The listing builds one solid part. Answer for the finished solid, in the listing's coordinates (mm). A direction names the side the tool comes from. Round coordinates to 2 decimals unless told otherwise and drop trailing zeros. Loops run counter-clockwise (first coordinate to the right, second up) from the corner with the lowest first, then second, coordinate; pieces in that order, holes last. Notation, with made-up numbers: (12.25, 41.25) -> (57.25, 41.25) arc R15 ccw to (57.25, 50.25) -> close; hole circle Ø11 at (-33, 11). An arc over 180 degrees is marked (long way). Use a Markdown table: item, result. Add a question column.
Q1. Consider line 1 (X direction, y = 0.5, z = -180); line 2 (X direction, y = 2.4, z = -20); line 3 (X direction, y = 1.65, z = -105). Determine where each line is inside the solid, lowest interval first.
Q2. Section C-C on x = 42.5 is taken. Give the vertices of the cut face in (y, z), then the cut area to 3 significant figures.
Q3. Section D-D on y = -1.5 is taken. Give the vertices of the cut face in (x, z), then the cut area to 3 significant figures.
Q4. Section A-A on z = -132.5 is taken. Give the vertices of the cut face in (x, y).
Q5. For a pull along X with two mould halves and no side action, classify faces 1 (the flat face through (0, 2, -96)), 2 (the cylindrical face through (117.6, 2, -170)) as released by +X, released by -X, zero draft, split by the parting line, or undercut.
Q6. Which of the six approach directions +Z, -Z, +X, -X, +Y, -Y give full straight-line access (tool end or side, diameter ignored) to faces 3 (the cylindrical face through (10, 2, -150)), 4 (the cylindrical face through (165, 2, -10))?
Q7. Given pin 1 Ø2 at (x, y) = (136, -2) entering from -Z, flat-ended and moving along its own axis, determine where the tip first touches the part or whether it passes through.
Q8. Section B-B on x = 115 is taken. Give the vertices of the cut face in (y, z).
from build123d import *

# Parameters (mm, degrees)
SKETCH1_W           = 200
SKETCH1_H           = 190
BOSS_EXTRUDE1_DEPTH = 4
SKETCH3_R           = 50
CUT_EXTRUDE5_DEPTH  = 10
SKETCH4_W           = 200
SKETCH4_H           = 4
BOSS_EXTRUDE2_DEPTH = 4
SKETCH_1_R          = 8
CUT_EXTRUDE_1_DEPTH = 10


with BuildPart() as part:
    # Sketch1 → Boss-Extrude1 (new body)
    with BuildSketch(Plane(origin=(0, 0, 0), x_dir=(1, 0, 0), z_dir=(0, 1, 0))):
        with Locations((100, 95)):
            Rectangle(SKETCH1_W, SKETCH1_H)
    extrude(amount=BOSS_EXTRUDE1_DEPTH)

    # Sketch3 → Cut-Extrude5 (cut)
    with BuildSketch(Plane(origin=(0, 4, 0), x_dir=(1, 0, 0), z_dir=(0, 1, 0))):
        with BuildLine():
            Line((30, 15), (20.262068061, 15))
            ThreePointArc((20.262068061, 15), (16.735494747, 16.716132106), (15, 20.233217082))
            Line((15, 20.233217082), (15, 30))
            ThreePointArc((15, 30), (10, 35), (5, 30))
            Line((5, 30), (5, 20.194837008))
            ThreePointArc((5, 20.194837008), (4.997925704, 19.868737095), (5.017113168, 19.54319555))
            ThreePointArc((5.017113168, 19.54319555), (9.654794827, 9.654664453), (19.545086076, 5.020737673))
            ThreePointArc((19.545086076, 5.020737673), (19.772306824, 5.005187109), (20, 5))
            Line((20, 5), (30, 5))
            ThreePointArc((30, 5), (35, 10), (30, 15))
        make_face()
        with BuildLine():
            Line((5, 90), (5, 50))
            ThreePointArc((5, 50), (10, 45), (15, 50))
            Line((15, 50), (15, 90))
            ThreePointArc((15, 90), (10, 95), (5, 90))
        make_face()
        with BuildLine():
            Line((70, 15), (50, 15))
            ThreePointArc((50, 15), (45, 10), (50, 5))
            Line((50, 5), (70, 5))
            ThreePointArc((70, 5), (75, 10), (70, 15))
        make_face()
        with BuildLine():
            ThreePointArc((185, 50), (190, 45), (195, 50))
            Line((195, 50), (195, 90))
            ThreePointArc((195, 90), (190, 95), (185, 90))
            Line((185, 90), (185, 50))
        make_face()
        with BuildLine():
            ThreePointArc((185, 20.233217082), (183.264505253, 16.716132106), (179.737931939, 15))
            Line((179.737931939, 15), (170, 15))
            ThreePointArc((170, 15), (165, 10), (170, 5))
            Line((170, 5), (180, 5))
            ThreePointArc((180, 5), (180.227693176, 5.005187109), (180.454913924, 5.020737673))
            ThreePointArc((180.454913924, 5.020737673), (190.345205173, 9.654664453), (194.982886832, 19.54319555))
            ThreePointArc((194.982886832, 19.54319555), (195.002074296, 19.868737095), (195, 20.194837008))
            Line((195, 20.194837008), (195, 30))
            ThreePointArc((195, 30), (190, 35), (185, 30))
            Line((185, 30), (185, 20.233217082))
        make_face()
        with BuildLine():
            ThreePointArc((150, 5), (155, 10), (150, 15))
            Line((150, 15), (130, 15))
            ThreePointArc((130, 15), (125, 10), (130, 5))
            Line((130, 5), (150, 5))
        make_face()
        with BuildLine():
            ThreePointArc((160.821819194, 46.262953407), (161.237046593, 53.321819194), (154.178180806, 53.737046593))
            Line((154.178180806, 53.737046593), (131.678180806, 33.737046593))
            ThreePointArc((131.678180806, 33.737046593), (131.262953407, 26.678180806), (138.321819194, 26.262953407))
            Line((138.321819194, 26.262953407), (160.821819194, 46.262953407))
        make_face()
        with BuildLine():
            Line((131.678180806, 156.262953407), (154.178180806, 136.262953407))
            ThreePointArc((154.178180806, 136.262953407), (161.237046593, 136.678180806), (160.821819194, 143.737046593))
            Line((160.821819194, 143.737046593), (138.321819194, 163.737046593))
            ThreePointArc((138.321819194, 163.737046593), (131.262953407, 163.321819194), (131.678180806, 156.262953407))
        make_face()
        with BuildLine():
            Line((5.5, 135), (5.5, 120))
            ThreePointArc((5.5, 120), (10, 115.5), (14.5, 120))
            Line((14.5, 120), (14.5, 135))
            ThreePointArc((14.5, 135), (10, 139.5), (5.5, 135))
        make_face()
        with BuildLine():
            ThreePointArc((39.178180806, 143.737046593), (38.762953407, 136.678180806), (45.821819194, 136.262953407))
            Line((45.821819194, 136.262953407), (68.321819194, 156.262953407))
            ThreePointArc((68.321819194, 156.262953407), (68.737046593, 163.321819194), (61.678180806, 163.737046593))
            Line((61.678180806, 163.737046593), (39.178180806, 143.737046593))
        make_face()
        with BuildLine():
            Line((68.321819194, 33.737046593), (45.821819194, 53.737046593))
            ThreePointArc((45.821819194, 53.737046593), (38.762953407, 53.321819194), (39.178180806, 46.262953407))
            Line((39.178180806, 46.262953407), (61.678180806, 26.262953407))
            ThreePointArc((61.678180806, 26.262953407), (68.737046593, 26.678180806), (68.321819194, 33.737046593))
        make_face()
        with BuildLine():
            Line((95, 190), (95, 170))
            ThreePointArc((95, 170), (100, 165), (105, 170))
            Line((105, 170), (105, 190))
            ThreePointArc((105, 190), (100, 195), (95, 190))
        make_face()
        with BuildLine():
            Line((77.335483589, 190), (77.335483589, 175))
            ThreePointArc((77.335483589, 175), (82.335483589, 170), (87.335483589, 175))
            Line((87.335483589, 175), (87.335483589, 190))
            ThreePointArc((87.335483589, 190), (82.335483589, 195), (77.335483589, 190))
        make_face()
        with BuildLine():
            Line((5, 207.20463147), (5, 155))
            ThreePointArc((5, 155), (10, 150), (15, 155))
            Line((15, 155), (15, 207.20463147))
            ThreePointArc((15, 207.20463147), (10, 212.20463147), (5, 207.20463147))
        make_face()
        with BuildLine():
            ThreePointArc((185, 155), (190, 150), (195, 155))
            Line((195, 155), (195, 207.20463147))
            ThreePointArc((195, 207.20463147), (190, 212.20463147), (185, 207.20463147))
            Line((185, 207.20463147), (185, 155))
        make_face()
        with BuildLine():
            ThreePointArc((112.664516411, 175), (117.664516411, 170), (122.664516411, 175))
            Line((122.664516411, 175), (122.664516411, 190))
            ThreePointArc((122.664516411, 190), (117.664516411, 195), (112.664516411, 190))
            Line((112.664516411, 190), (112.664516411, 175))
        make_face()
        with BuildLine():
            ThreePointArc((185.5, 120), (190, 115.5), (194.5, 120))
            Line((194.5, 120), (194.5, 135))
            ThreePointArc((194.5, 135), (190, 139.5), (185.5, 135))
            Line((185.5, 135), (185.5, 120))
        make_face()
        with Locations(Location((100, 95, 0), (0, 0, 270))):
            Circle(SKETCH3_R)
    extrude(amount=-CUT_EXTRUDE5_DEPTH, mode=Mode.SUBTRACT)

    # Sketch4 → Boss-Extrude2 (add)
    with BuildSketch(Plane.XZ):
        with Locations((100, -2)):
            Rectangle(SKETCH4_W, SKETCH4_H)
    extrude(amount=BOSS_EXTRUDE2_DEPTH)

    # Sketch 1 → Cut-Extrude 1 (cut)
    with BuildSketch(Plane(origin=(0, 4, 0), x_dir=(1, 0, 0), z_dir=(0, 1, 0))):
        with Locations(Location((100, 20, 0), (0, 0, 270))):
            Circle(SKETCH_1_R)
        with Locations(Location((190, 105, 0), (0, 0, 270))):
            Circle(SKETCH_1_R)
        with Locations(Location((10, 105, 0), (0, 0, 270))):
            Circle(SKETCH_1_R)
    extrude(amount=-CUT_EXTRUDE_1_DEPTH, mode=Mode.SUBTRACT)


solid = part.part
Checked values:
| question | item | result |
|---|---|---|
| 1 | line 1 | x = 0 to 5, 15 to 77.34, 87.34 to 95, 105 to 112.66, 122.66 to 185, 195 to 200 |
| 1 | line 2 | x = 0 to 5, 15.03 to 92, 108 to 184.97, 195 to 200 |
| 1 | line 3 | x = 0 to 2, 18 to 51.01, 148.99 to 182, 198 to 200 |
| 2 | outline | (-4, -4) -> (0, -4) -> (0, -43.31) -> (4, -43.31) -> (4, 0) -> (-4, 0) -> close; (0, -190) -> (4, -190) -> (4, -146.69) -> (0, -146.69) -> close; (0, -135) -> (4, -135) -> (4, -55) -> (0, -55) -> close |
| 2 | area | 682 mm2 |
| 3 | outline | (0, -4) -> (200, -4) -> (200, 0) -> (0, 0) -> close |
| 3 | area | 800 mm2 |
| 4 | outline | (0, 0) -> (5.5, 0) -> (5.5, 4) -> (0, 4) -> close; (14.5, 0) -> (66.93, 0) -> (66.93, 4) -> (14.5, 4) -> close; (133.07, 0) -> (185.5, 0) -> (185.5, 4) -> (133.07, 4) -> close; (194.5, 0) -> (200, 0) -> (200, 4) -> (194.5, 4) -> close |
| 5 | face 1 | released by -X |
| 5 | face 2 | undercut |
| 6 | face 3 | -Z, +Y, -Y |
| 6 | face 4 | +Y, -Y |
| 7 | pin 1 | stops at z = -4 |
| 8 | outline | (-4, -4) -> (0, -4) -> (0, -47.3) -> (4, -47.3) -> (4, 0) -> (-4, 0) -> close; (0, -170.77) -> (4, -170.77) -> (4, -142.7) -> (0, -142.7) -> close |
